from build123d import *

# Parameters (mm, degrees)
SKETCH1_R      = 2.5
EXTRUDE1_DEPTH = 9


# Read off the part's stored shape, not the designer's step: Cut-Extrude1
with BuildPart() as part:
    # Sketch1 → Extrude1 (new, symmetric)
    with BuildSketch(Plane(origin=(0, 0, 0), x_dir=(0, 0, -1), z_dir=(1, 0, 0))):
        Polygon((5.773502692, 0), (2.886751346, 5), (-2.886751346, 5), (-5.773502692, 0), (-2.886751346, -5), (2.886751346, -5), align=None)
        Circle(SKETCH1_R, mode=Mode.SUBTRACT)
    extrude(amount=EXTRUDE1_DEPTH, both=True)

    # Cut-Extrude1 outline → Cut-Extrude1 (revolve, cut)
    with BuildSketch(Plane.YX):
        Polygon((5.773502692, 9.000000845), (4.99999886, 9.000000845), (5.773502688, 8.553418015), align=None)
    cut_extrude1 = revolve(axis=Axis((0, 0, 0), (1, 0, 0)), mode=Mode.SUBTRACT)

    # Mirror1: Cut-Extrude1 across plane
    add(cut_extrude1.mirror(Plane(origin=(0, 0, 0), x_dir=(0, 0, 1), z_dir=(1, 0, 0))), mode=Mode.SUBTRACT)


solid = part.part
The listing builds one solid part. Answer for the finished solid, in the listing's coordinates (mm). Coordinates: 2 decimals unless noted, no trailing zeros. Order: outer loops, then holes, each group sorted by start corner. A loop starts at its lowest first (then second) coordinate and runs counter-clockwise, first axis right, second up.
Q1. Consider line 1 (Y direction, x = 3, z = 0); line 2 (Z direction, x = 8, y = 1.75); line 3 (Z direction, x = 0.5, y = -2). Determine where each line is inside the solid, lowest interval first.
Q2. A cutting plane is placed at A-A, the plane x = 0.75. Write down the section's boundary in (y, z), and give its area (3 significant figures).
Q3. For a pull along Y with two mould halves and no side action, classify faces 1 (the face through (0, -5, 0)), 2 (the face through (-0.13, -2.44, 0.54)), 3 (the face through (-9, -2, -2)), 4 (the face through (8.89, 4.49, -2.61)) as pulls with the +Y half, pulls with the -Y half, needs draft (parallel to the pull), parting line crosses it, or undercut.
Q4. Given P1, Ø5, axis at x = -3.5, y = 3, coming from the +Z side; P2, Ø2, axis at x = 6, y = 3, coming from the -Z side, each flat-ended and moving along its own axis, determine where each tip first touches the part or whether it passes through.
Answers follow:
1. line 1: y = -5 to -2.5, 2.5 to 5
1. line 2: z = -4.76 to -1.79, 1.79 to 4.76
1. line 3: z = -4.62 to -1.5, 1.5 to 4.62
2. outline: (-5, -2.89) - (0, -5.77) - (5, -2.89) - (5, 2.89) - (0, 5.77) - (-5, 2.89) - close; hole circle Ø5 at (0, 0)
2. area: 67.0 mm2
3. face 1: pulls with the -Y half
3. face 2: undercut
3. face 3: needs draft
3. face 4: pulls with the +Y half
4. P1: stops at z = 5.48
4. P2: stops at z = -4.62
